Could you check a few things on this model? Use its own coordinates, in mm. Face numbers are marked on the shaded views. A direction names the side the tool comes from. Coordinates: 2 decimals unless noted, no trailing zeros. Order: outer loops, then holes, each group sorted by start corner. A loop starts at its lowest first (then second) coordinate and runs counter-clockwise, first axis right, second up. Notation, with made-up numbers: (55.25, -11) -> (104.25, -11) arc R23 ccw to (104.25, 28) -> close; hole circle Ø1 at (5.5, -34.5). An arc over 180 degrees is marked (long way). Use a Markdown table: item, result. Add a question column.
1) If we section it at A-A (y = 0): Write out the boundary of the cut face in (x, z).
2) Will these pins go through, and if not, where does the flat tip stop? pin 1 Ø1 at (x, y) = (-7, -13.5) entering from +Z; pin 2 Ø4.5 at (x, y) = (-15, -16) entering from +Z; pin 3 Ø4 at (x, z) = (-14, 5) entering from +Y; pin 4 Ø3.5 at (x, y) = (-15.5, 15.5) entering from +Z.
3) If I drill on L1, parallel to Y at x = 0, z = 3.25; L2, parallel to Y at x = 0, z = -1; L3, parallel to Y at x = 7, z = -0.5, over which ranges is the centre line in solid material (lowest first)? Write a range as [from, to].
4) Thinking about a two-plate mould opening in Y: for the marked faces 4, 5 and 6, which applies, +Y half, -Y half, draft (parallel to the pull), parting line (faces both ways), or undercut?
5) Which directions (+Z, -Z, +X, -X, +Y, -Y) give clear straight access to the entire face, cutting with the end or side of a thin tool? Please do the marked faces 1, 2 and 3.
6) If we section it at B-B (z = 2): Write out the boundary of the cut face in (x, y), plus the area to 3 significant figures.
7) If we section it at D-D (x = -7): Write out the boundary of the cut face in (y, z), plus the area to 3 significant figures.
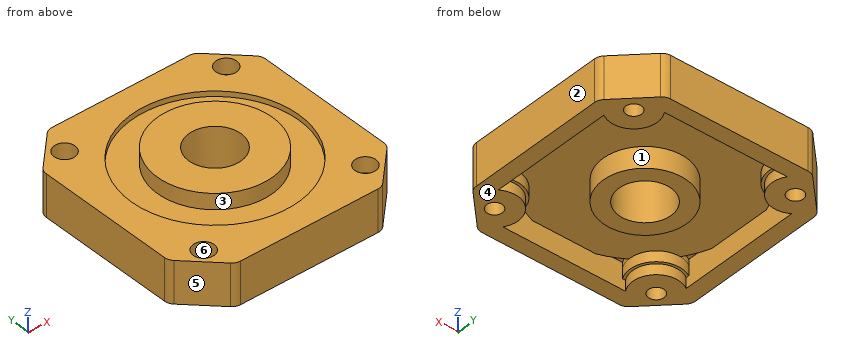
```python
from build123d import *

# Parameters (mm, degrees)
SKETCH1_W                               = 42
SKETCH1_H                               = 42
BOSS_EXTRUDE1_DEPTH                     = 4
CUT_EXTRUDE1_REACH                      = 32.757
SKETCH3_R                               = 16
SKETCH3_R_2                             = 11
CUT_EXTRUDE2_DEPTH                      = 1
BOSS_EXTRUDE2_START                     = 2
SKETCH4_R                               = 11
BOSS_EXTRUDE2_DEPTH                     = 2
CUT_EXTRUDE3_REACH                      = 33.337
SKETCH5_R                               = 5
CBORE_FOR_M5_HEX_HEAD_BOLT2_D           = 3
CBORE_FOR_M5_HEX_HEAD_BOLT2_DEPTH       = 10
CBORE_FOR_M5_HEX_HEAD_BOLT2_CBORE_D     = 4
CBORE_FOR_M5_HEX_HEAD_BOLT2_CBORE_DEPTH = 3
CBORE_FOR_M5_HEX_HEAD_BOLT2_TIP         = 0.901290929
SHELL1_START                            = -4
SHELL1_OUTLINE_R                        = 8
SHELL1_DEPTH                            = 4
SHELL1_2_DEPTH                          = 2
SHELL1_3_DEPTH                          = 1
FILLET1_R                               = 2


# Read off the part's stored shape, not the designer's step: Shell1
with BuildPart() as part:
    # Sketch1 → Boss-Extrude1 (new, symmetric)
    with BuildSketch(Plane.XY):
        Rectangle(SKETCH1_W, SKETCH1_H)
    extrude(amount=BOSS_EXTRUDE1_DEPTH, both=True)

    # Sketch2 → Cut-Extrude1 (cut, up to next)
    with BuildSketch(Plane.XY.offset(4), mode=Mode.PRIVATE) as cut_extrude1_sk1:
        Polygon((-21, 21), (-21, 14), (-14, 21), align=None)
    cut_extrude1_tool1 = extrude(cut_extrude1_sk1.sketch, amount=-CUT_EXTRUDE1_REACH, mode=Mode.PRIVATE) & part.part
    # Sketch2 → Cut-Extrude1 (cut, up to next)
    with BuildSketch(Plane.XY.offset(4), mode=Mode.PRIVATE) as cut_extrude1_sk2:
        Polygon((21, 14), (14, 21), (21, 21), align=None)
    cut_extrude1_tool2 = extrude(cut_extrude1_sk2.sketch, amount=-CUT_EXTRUDE1_REACH, mode=Mode.PRIVATE) & part.part
    # Sketch2 → Cut-Extrude1 (cut, up to next)
    with BuildSketch(Plane.XY.offset(4), mode=Mode.PRIVATE) as cut_extrude1_sk3:
        Polygon((21, -21), (21, -14), (14, -21), align=None)
    cut_extrude1_tool3 = extrude(cut_extrude1_sk3.sketch, amount=-CUT_EXTRUDE1_REACH, mode=Mode.PRIVATE) & part.part
    # Sketch2 → Cut-Extrude1 (cut, up to next)
    with BuildSketch(Plane.XY.offset(4), mode=Mode.PRIVATE) as cut_extrude1_sk4:
        Polygon((-21, -14), (-14, -21), (-21, -21), align=None)
    cut_extrude1_tool4 = extrude(cut_extrude1_sk4.sketch, amount=-CUT_EXTRUDE1_REACH, mode=Mode.PRIVATE) & part.part
    add(cut_extrude1_tool1.solids().sort_by_distance((-18.666667, 18.666667, 4))[0], mode=Mode.SUBTRACT)
    add(cut_extrude1_tool2.solids().sort_by_distance((18.666667, 18.666667, 4))[0], mode=Mode.SUBTRACT)
    add(cut_extrude1_tool3.solids().sort_by_distance((18.666667, -18.666667, 4))[0], mode=Mode.SUBTRACT)
    add(cut_extrude1_tool4.solids().sort_by_distance((-18.666667, -18.666667, 4))[0], mode=Mode.SUBTRACT)

    # Sketch3 → Cut-Extrude2 (cut)
    with BuildSketch(Plane.XY.offset(4)):
        Circle(SKETCH3_R)
        Circle(SKETCH3_R_2, mode=Mode.SUBTRACT)
    extrude(amount=-CUT_EXTRUDE2_DEPTH, mode=Mode.SUBTRACT)

    # Sketch4 → Boss-Extrude2 (add)
    with BuildSketch(Plane.XY.offset(4).offset(BOSS_EXTRUDE2_START)):
        Circle(SKETCH4_R)
    extrude(amount=-BOSS_EXTRUDE2_DEPTH)

    # Sketch5 → Cut-Extrude3 (cut, up to next)
    with BuildSketch(Plane.XY.offset(6), mode=Mode.PRIVATE) as cut_extrude3_sk1:
        Circle(SKETCH5_R)
    cut_extrude3_tool1 = extrude(cut_extrude3_sk1.sketch, amount=-CUT_EXTRUDE3_REACH, mode=Mode.PRIVATE) & part.part
    add(cut_extrude3_tool1.solids().sort_by_distance((0, 0, 6))[0], mode=Mode.SUBTRACT)

    # CBORE for M5 Hex Head Bolt2
    with Locations(Plane.XY.offset(4)):
        with Locations((-15.5, 15.5), (15.5, 15.5), (15.5, -15.5), (-15.5, -15.5)):
            CounterBoreHole(CBORE_FOR_M5_HEX_HEAD_BOLT2_D / 2, CBORE_FOR_M5_HEX_HEAD_BOLT2_CBORE_D / 2, CBORE_FOR_M5_HEX_HEAD_BOLT2_CBORE_DEPTH, depth=CBORE_FOR_M5_HEX_HEAD_BOLT2_DEPTH)
            with Locations((0, 0, -(CBORE_FOR_M5_HEX_HEAD_BOLT2_DEPTH + CBORE_FOR_M5_HEX_HEAD_BOLT2_TIP / 2))):  # 118° drill point
                Cone(0, CBORE_FOR_M5_HEX_HEAD_BOLT2_D / 2, CBORE_FOR_M5_HEX_HEAD_BOLT2_TIP, mode=Mode.SUBTRACT)

    # Shell1 outline → Shell1 (cut)
    with BuildSketch(Plane.XY.offset(SHELL1_START)):
        with BuildLine():
            ThreePointArc((-18, -11.169872981), (-11.964466094, -11.964466094), (-11.169872981, -18))
            Line((-11.169872981, -18), (11.169872981, -18))
            ThreePointArc((11.169872981, -18), (11.964466094, -11.964466094), (18, -11.169872981))
            Line((18, -11.169872981), (18, 11.169872981))
            ThreePointArc((18, 11.169872981), (11.964466094, 11.964466094), (11.169872981, 18))
            Line((11.169872981, 18), (-11.169872981, 18))
            ThreePointArc((-11.169872981, 18), (-11.964466094, 11.964466094), (-18, 11.169872981))
            Line((-18, 11.169872981), (-18, -11.169872981))
        make_face()
        Circle(SHELL1_OUTLINE_R, mode=Mode.SUBTRACT)
    extrude(amount=SHELL1_DEPTH, mode=Mode.SUBTRACT)

    # Shell1 2 outline → Shell1 2 (cut)
    with BuildSketch(Plane.XY.offset(SHELL1_START)):
        with BuildLine():
            Line((-18, -11.169872981), (-18, -11.758342613))
            ThreePointArc((-18, -11.758342613), (-12.318019485, -12.318019485), (-11.758342613, -18))
            Line((-11.758342613, -18), (-11.169872981, -18))
            ThreePointArc((-11.169872981, -18), (-11.964466094, -11.964466094), (-18, -11.169872981))
        make_face()
        with BuildLine():
            Line((-18, 11.758342613), (-18, 11.169872981))
            ThreePointArc((-18, 11.169872981), (-11.964466094, 11.964466094), (-11.169872981, 18))
            Line((-11.169872981, 18), (-11.758342613, 18))
            ThreePointArc((-11.758342613, 18), (-12.318019485, 12.318019485), (-18, 11.758342613))
        make_face()
        with BuildLine():
            ThreePointArc((18, -11.169872981), (11.964466094, -11.964466094), (11.169872981, -18))
            Line((11.169872981, -18), (11.758342613, -18))
            ThreePointArc((11.758342613, -18), (12.318019485, -12.318019485), (18, -11.758342613))
            Line((18, -11.758342613), (18, -11.169872981))
        make_face()
        with BuildLine():
            Line((11.758342613, 18), (11.169872981, 18))
            ThreePointArc((11.169872981, 18), (11.964466094, 11.964466094), (18, 11.169872981))
            Line((18, 11.169872981), (18, 11.758342613))
            ThreePointArc((18, 11.758342613), (12.318019485, 12.318019485), (11.758342613, 18))
        make_face()
    extrude(amount=SHELL1_2_DEPTH, mode=Mode.SUBTRACT)

    # Shell1 3 outline → Shell1 3 (cut)
    with BuildSketch(Plane.XY):
        with BuildLine():
            Line((-18, -6.08276253), (-18, -11.169872981))
            ThreePointArc((-18, -11.169872981), (-16.951868237, -10.715433288), (-15.827943399, -10.510766278))
            ThreePointArc((-15.827943399, -10.510766278), (-17.058260256, -8.367541876), (-18, -6.08276253))
        make_face()
        with BuildLine():
            ThreePointArc((-10.510766278, -15.827943399), (-10.715433288, -16.951868237), (-11.169872981, -18))
            Line((-11.169872981, -18), (-6.08276253, -18))
            ThreePointArc((-6.08276253, -18), (-8.367541876, -17.058260256), (-10.510766278, -15.827943399))
        make_face()
        with BuildLine():
            Line((-18, 11.169872981), (-18, 6.08276253))
            ThreePointArc((-18, 6.08276253), (-17.058260256, 8.367541876), (-15.827943399, 10.510766279))
            ThreePointArc((-15.827943399, 10.510766279), (-16.951868237, 10.715433288), (-18, 11.169872981))
        make_face()
        with BuildLine():
            ThreePointArc((10.510766279, -15.827943399), (8.367541876, -17.058260256), (6.08276253, -18))
            Line((6.08276253, -18), (11.169872981, -18))
            ThreePointArc((11.169872981, -18), (10.715433288, -16.951868237), (10.510766279, -15.827943399))
        make_face()
        with BuildLine():
            ThreePointArc((-11.169872981, 18), (-10.715433288, 16.951868237), (-10.510766278, 15.827943399))
            ThreePointArc((-10.510766278, 15.827943399), (-8.367541876, 17.058260256), (-6.08276253, 18))
            Line((-6.08276253, 18), (-11.169872981, 18))
        make_face()
        with BuildLine():
            ThreePointArc((18, -6.08276253), (17.058260256, -8.367541876), (15.827943399, -10.510766279))
            ThreePointArc((15.827943399, -10.510766279), (16.951868237, -10.715433288), (18, -11.169872981))
            Line((18, -11.169872981), (18, -6.08276253))
        make_face()
        with BuildLine():
            Line((11.169872981, 18), (6.08276253, 18))
            ThreePointArc((6.08276253, 18), (8.367541876, 17.058260256), (10.510766279, 15.827943399))
            ThreePointArc((10.510766279, 15.827943399), (10.715433288, 16.951868237), (11.169872981, 18))
        make_face()
        with BuildLine():
            ThreePointArc((15.827943399, 10.510766279), (17.058260256, 8.367541876), (18, 6.08276253))
            Line((18, 6.08276253), (18, 11.169872981))
            ThreePointArc((18, 11.169872981), (16.951868237, 10.715433288), (15.827943399, 10.510766279))
        make_face()
    extrude(amount=SHELL1_3_DEPTH, mode=Mode.SUBTRACT)

    # Fillet1
    fillet1_edges = [part.edges().sort_by_distance(p)[0] for p in [
        (-21, -14, 0),
        (-14, -21, 0),
        (14, -21, 0),
        (21, -14, 0),
        (21, 14, 0),
        (14, 21, 0),
        (-14, 21, 0),
        (-21, 14, 0),
    ]]
    fillet(fillet1_edges, radius=FILLET1_R)


solid = part.part
```
Answer sheet:
| question | item | result |
|---|---|---|
| 1 | outline | (-21, -4) -> (-18, -4) -> (-18, 0) -> (-8, 0) -> (-8, -4) -> (-5, -4) -> (-5, 6) -> (-11, 6) -> (-11, 3) -> (-16, 3) -> (-16, 4) -> (-21, 4) -> close; (5, -4) -> (8, -4) -> (8, 0) -> (18, 0) -> (18, -4) -> (21, -4) -> (21, 4) -> (16, 4) -> (16, 3) -> (11, 3) -> (11, 6) -> (5, 6) -> close |
| 2 | pin 1 | z = 3 |
| 2 | pin 2 | z = 4 |
| 2 | pin 3 | y = 21 |
| 2 | pin 4 | z = 1 |
| 3 | L1 | [-21, -16], [-11, -5], [5, 11], [16, 21] |
| 3 | L2 | [-21, -18], [-8, -5], [5, 8], [18, 21] |
| 3 | L3 | [-21, -18], [-3.87, 3.87], [18, 21] |
| 4 | face 4 | draft |
| 4 | face 5 | -Y half |
| 4 | face 6 | undercut |
| 5 | face 1 | -Z |
| 5 | face 2 | +Z, -Z, +X, +Y, -Y |
| 5 | face 3 | +Z |
| 6 | outline | (-21, -13.17) arc R2 ccw to (-20.41, -14.59) -> (-14.59, -20.41) arc R2 ccw to (-13.17, -21) -> (13.17, -21) arc R2 ccw to (14.59, -20.41) -> (20.41, -14.59) arc R2 ccw to (21, -13.17) -> (21, 13.17) arc R2 ccw to (20.41, 14.59) -> (14.59, 20.41) arc R2 ccw to (13.17, 21) -> (-13.17, 21) arc R2 ccw to (-14.59, 20.41) -> (-20.41, 14.59) arc R2 ccw to (-21, 13.17) -> close; hole circle Ø4 at (-15.5, -15.5); hole circle Ø4 at (-15.5, 15.5); hole circle Ø10 at (0, 0); hole circle Ø4 at (15.5, -15.5); hole circle Ø4 at (15.5, 15.5) |
| 6 | area | 1,540 mm2 |
| 7 | outline | (-21, -4) -> (-18, -4) -> (-18, 1) -> (-17.66, 1) -> (-17.66, 0) -> (-3.87, 0) -> (-3.87, -4) -> (3.87, -4) -> (3.87, 0) -> (17.66, 0) -> (17.66, 1) -> (18, 1) -> (18, -4) -> (21, -4) -> (21, 4) -> (14.39, 4) -> (14.39, 3) -> (8.49, 3) -> (8.49, 6) -> (-8.49, 6) -> (-8.49, 3) -> (-14.39, 3) -> (-14.39, 4) -> (-21, 4) -> close |
| 7 | area | 244 mm2 |
